Autodesk Inventor part; units mm, degrees
ref_plane "YZ Plane" through (0, 0, 0) normal (1, 0, 0) x (0, 1, 0)
ref_plane "XZ Plane" through (0, 0, 0) normal (0, 1, 0) x (-1, 0, 0)
ref_plane "XY Plane" through (0, 0, 0) normal (0, 0, 1) x (1, 0, 0)
sketch "Sketch1" plane through (0, 0, 0) normal (0, 1, 0) x (-1, 0, 0)
  arc A0 (-93.5462, 17.5) -> (-93.5462, -17.5) centre (-93.5462, 0) ccw
  arc A1 (-93.5462, 17.5) -> (-93.5462, -17.5) centre (-93.5462, 0) ccw
  line L0 (-68.5462, -17.5) -> (51.4538, -17.5)
  line L1 (51.4538, -17.5) -> (51.4538, 12.6842)
  line L2 (51.4538, 12.6842) -> (-68.5462, 12.6842)
  line L3 (-68.5462, 12.6842) -> (-68.5462, -17.5)
  line L4 (-68.5462, -17.5) -> (-93.5462, -17.5)
  arc A2 (76.4538, -17.5) -> (76.4538, 17.5) centre (76.4538, 0) ccw
  line L5 (51.4538, -17.5) -> (76.4538, -17.5)
  line L6 (76.4538, 17.5) -> (-93.5462, 17.5)
  point P0 (0, 0)
  dimension "d0" = 35
  dimension "d1" = 120
  dimension "d2" = 25
  dimension "d3" = 35
  dimension "d4" = 25
extrude "Extrusion1" add sketch "Sketch1" along normal blind 65 contours L6 A2 L5 L1 L2 L3 L4 A0
sketch "Sketch2" plane through (0, 65, 0) normal (0, 1, 0) x (1, 0, 0)
  arc A0 (-69.3673, -11.4905) -> (-75.5737, -13.4713) centre (-76.4538, 0) ccw
  arc A1 (92.6661, -13.4713) -> (86.972, -11.7911) centre (93.5462, 0) ccw
  line L0 (-51.4538, -12.6842) -> (-51.4538, 17.5)
  line L1 (68.5462, 17.5) -> (68.5462, -12.6842)
  line L2 (93.5462, -13.5) -> (68.5462, -12.6842)
  line L3 (-76.4538, -13.5) -> (-51.4538, -12.6842)
  line L4 (68.5462, -11.1899) -> (86.972, -11.7911)
  line L5 (-51.4538, -11.8536) -> (-69.3673, -11.4905)
  line L6 (-51.4538, -11.8536) -> (-51.4267, -12.6833)
  line L7 (68.5462, -11.1899) -> (68.5462, -12.6842)
  point P0 (0, 0)
  dimension "d7" = 27
  dimension "d8" = 27
  dimension "d9" = 25
  dimension "d10" = 25
extrude "Extrusion2" cut sketch "Sketch2" against normal blind 65 contours L5 L0 L3 A0 | L2 L1 L4 A1
sketch "Sketch4" plane through (0, 0, 0) normal (0, -1, 0) x (1, 0, 0)
  arc A0 (-76.4538, 13.5) -> (-69.3673, 11.4905) centre (-76.4538, 0) ccw
  arc A1 (-76.4538, 17.5) -> (-76.4538, -17.5) centre (-76.4538, 0) ccw
  arc A2 (93.5462, -17.5) -> (93.5462, 17.5) centre (93.5462, 0) ccw
  arc A3 (93.5462, -17.5) -> (93.5462, 17.5) centre (93.5462, 0) ccw
  line L0 (-76.4538, 17.5) -> (93.5462, 17.5)
  line L1 (-76.4538, 17.5) -> (93.5462, 17.5)
  line L2 (-51.4538, -17.5) -> (-76.4538, -17.5)
  line L3 (-76.4538, -17.5) -> (93.5462, -17.5)
  point P0 (0, 0)
extrude "Extrusion4" add sketch "Sketch4" along normal blind 5
sketch "Sketch5" plane through (0, 0, 0) normal (0, 1, 0) x (1, 0, 0)
  line L0 (-69.3673, -11.4905) -> (-51.4538, -11.8536)
  line L1 (68.5462, 17.5) -> (68.5462, -11.1899)
  line L2 (-51.4538, -11.8536) -> (68.5462, -11.8536)
  line L3 (68.5462, -11.8536) -> (68.5462, -8.8458)
  line L4 (68.5462, -8.8458) -> (-51.4538, -8.8458)
  line L5 (-51.4538, -8.8458) -> (-51.4538, -11.8536)
  point P0 (0, 0)
extrude "Extrusion5" add sketch "Sketch5" along normal blind 2
sketch "Sketch6" plane through (68.5462, 0, 8.8458) normal (0, 0, -1) x (-1, 0, 0)
  point P0 (68.5462, 0)
sketch "Sketch7" plane through (0, 0, 0) normal (0, 1, 0) x (1, 0, 0)
  line L0 (68.5462, -11.8536) -> (68.5462, -11.1899)
  line L1 (68.5462, -11.1899) -> (86.972, -11.7911)
  line L2 (68.5462, -11.8536) -> (86.972, -11.7911)
  line L3 (68.5462, -8.8458) -> (68.5462, -11.1899)
  line L4 (86.972, -11.7911) -> (68.5462, -11.1899)
  line L5 (68.5462, -11.1899) -> (68.5266, -11.7911)
  point P0 (0, 0)
extrude "Extrusion6" add sketch "Sketch7" along normal blind 65
sketch "Sketch8" plane through (-51.4538, 65, 11.8536) normal (1, 0, 0) x (0, 0, -1)
  line L0 (0, 0) -> (29.3536, 0)
  line L1 (0, 0) -> (4.0071, 0)
  line L2 (4.0071, 0) -> (4.0071, -2.0911)
  line L3 (4.0071, -2.0911) -> (0, -2.0911)
  line L4 (0, -2.0911) -> (0, 0)
  point P0 (11.8536, -65)
extrude "Extrusion7" add sketch "Sketch8" along normal blind 120
fillet "Fillet1" radius 0.5 1 edges at (-69.3673, 32.5, 11.4905)
fillet "Fillet2" radius 0.5 1 edges at (86.972, 32.5, 11.7911)
chamfer "Chamfer1" distance 1 angle 45 1 edges at (8.5462, 2, 8.8458)
chamfer "Chamfer2" distance 1 angle 45 1 edges at (8.5462, 62.9089, 7.8466)
sketch "Sketch9" plane through (0, 0, 0) normal (0, 1, 0) x (1, 0, 0)
  arc A0 (93.5462, -17.5) -> (93.5462, 17.5) centre (93.5462, 0) ccw
  line L0 (93.5462, 17.5) -> (68.5462, 17.5)
  line L1 (93.5462, 17.5) -> (93.5462, 17.5)
  circle A1 centre (93.5462, 0) radius 2
  line L2 (-76.4538, 17.5) -> (93.5462, 17.5)
  line L3 (-76.4538, -17.5) -> (93.5462, -17.5)
  circle A2 centre (-76.4538, 0) radius 2
  point P0 (0, 0)
  dimension "d39" = 4
  dimension "d40" = 4
extrude "Extrusion8" add sketch "Sketch9" along normal blind 5
fillet "Fillet3" radius 0.5 2 edges at (91.5462, 5, 0) (-78.4538, 5, 0)
sketch "Sketch10" plane through (-51.4538, 65, -17.5) normal (0, 0, -1) x (-1, 0, 0)
  circle A0 centre (-125, -5) radius 1.75
  circle A1 centre (-125, -60) radius 1.75
  line L0 (25, -70) -> (-145, -70)
  line L1 (-120, -65) -> (-120, 0)
  line L2 (-145, 0) -> (-120, 0)
  circle A2 centre (5, -60) radius 1.75
  circle A3 centre (5, -5) radius 1.75
  line L3 (0, -65) -> (0, 0)
  line L4 (0, 0) -> (25, 0)
  point P0 (-51.4538, -65)
  dimension "d44" = 3.5
  dimension "d45" = 3.5
  dimension "d46" = 10
  dimension "d47" = 5
  dimension "d48" = 5
  dimension "d49" = 3.5
  dimension "d50" = 3.5
  dimension "d51" = 5
  dimension "d52" = 5
  dimension "d53" = 5
  dimension "d54" = 10
extrude "Extrusion9" cut sketch "Sketch10" against normal blind 10
sketch "Sketch11" plane through (0, 65, 0) normal (0, 1, 0) x (1, 0, 0)
  point P0 (0, 0)
sketch "Sketch12" plane through (0, 65, 0) normal (0, 1, 0) x (1, 0, 0)
  circle A0 centre (73.5462, -2.5) radius 2
  circle A1 centre (-56.4538, -2.5) radius 2
  line L0 (68.5462, 17.5) -> (68.5462, -7.8466)
  line L1 (93.5462, 17.5) -> (68.5462, 17.5)
  line L2 (-51.4538, -7.8466) -> (-51.4538, 17.5)
  arc A2 (93.5462, -17.5) -> (93.5462, 17.5) centre (93.5462, 0) ccw
  point P0 (0, 0)
  dimension "d57" = 4
  dimension "d58" = 4
  dimension "d59" = 5
  dimension "d60" = 20
  dimension "d61" = 5
  dimension "d62" = 20
extrude "Extrusion10" cut sketch "Sketch12" against normal blind 10
sketch "Sketch13" plane through (0, 65, 0) normal (0, 1, 0) x (1, 0, 0)
  circle A0 centre (93.5462, 0) radius 1.5
  arc A1 (93.5462, -16.75) -> (93.5462, 16.75) centre (93.5462, 0) ccw
  circle A2 centre (93.5462, 0) radius 2
  arc A3 (93.5462, -15.75) -> (93.5462, 15.75) centre (93.5462, 0) ccw
  circle A4 centre (-76.4538, 0) radius 1.5
  arc A5 (-76.4538, 16.75) -> (-76.4538, -16.75) centre (-76.4538, 0) ccw
  arc A6 (-76.4538, 15.75) -> (-76.4538, -15.75) centre (-76.4538, 0) ccw
  line L0 (93.5462, -16.75) -> (-76.4538, -16.75)
  line L1 (-76.4538, -15.75) -> (93.5462, -15.75)
  line L2 (-76.4538, 15.75) -> (-55.2204, 15.75)
  line L3 (-55.2204, 15.75) -> (-55.2204, 16.75)
  line L4 (-55.2204, 16.75) -> (-76.4538, 16.75)
  line L5 (93.5462, 15.75) -> (71.4067, 15.75)
  line L6 (71.4067, 15.75) -> (71.4067, 16.75)
  line L7 (71.4067, 16.75) -> (93.5462, 16.75)
  point P0 (0, 0)
  dimension "d65" = 33.5
  dimension "d66" = 31.5
  dimension "d67" = 33.5
  dimension "d68" = 31.5
extrude "Extrusion11" add sketch "Sketch13" along normal blind 2 contours L0 A5 L4 L3 L2 A6 L1 A3 L5 L6 L7 A1
sketch "Sketch14" plane through (-51.4538, 65, -17.5) normal (0, 0, -1) x (-1, 0, 0)
  point P0 (-51.4538, -65)
properties part number "C-PAN"
The listing builds one solid part. Answer for the finished solid, in the listing's coordinates (mm). A direction names the side the tool comes from. Give positions to 0.01 mm unless a question says otherwise; leave off trailing zeros. Write each loop counter-clockwise with the first axis right and the second up, starting at its lowest first coordinate (ties: lowest second). Pieces come first, ordered by that corner, then holes. Notation, with made-up numbers: (48.5, 19.5) - (68.5, 19.5) arc R13 ccw to (68.5, 23.5) - close; hole circle Ø4 at (11, 63). An arc over 180 degrees is marked (long way). Use one line per item in the form item = value. Start each with the question number.
1) Find section A-A on x = 24.5. Determine the outline of the cut face in (y, z).
2) Find section D-D on x = 77.5. Determine the outline of the cut face in (y, z), plus the area to 3 significant figures.
3) The mould has two halves that part along X. Classify faces 1 (the face through (71.55, 60.07, 2.41)), 2 (the face through (-56, 5, -7.5)), 3 (the face through (-93.2, 66, 0.4)), 4 (the face through (9, -1, -17.5)): pulls with the +X half, pulls with the -X half, needs draft (parallel to the pull), parting line crosses it, or undercut.
4) Find section C-C on y = 12.5. Determine the outline of the cut face in (x, z).
5) Consider line 1 along Z through (x, y) = (-65, 60); line 2 along X through (y, z) = (32.5, -4); line 3 along Z through (x, y) = (-77, 24). Determine where each line is inside the solid, lowest interval first. Write a range as from..to.
6) Find section B-B on z = -11.5. Determine the outline of the cut face in (x, y).
7) Flat-ended cylindrical pins translate along their axes: pin 1 Ø1 at (y, z) = (16, -5) entering from -X; pin 2 Ø6 at (x, y) = (58, 40) entering from -Z; pin 3 Ø1.8 at (x, y) = (73, 60) entering from -Z; pin 4 Ø4.5 at (x, y) = (-56.45, 5) entering from -Z. Find the tip coordinate at first contact, or state that the pin passes through.
8) A tool of negligible diameter and unlimited length cuts with its end or side. For faces 5 (the face through (73.926, 3.292, -12.57)), 6 (the face through (-93.95, 30.49, -0.38)), 7 (the face through (-92.2, 66, 0.3)), from which of +Z, -Z, +X, -X, +Y, -Y can it reach the whole face along a straight path? Write none if from no direction.
Geometry results:
q1.outline = (-5, -17.5) - (0, -17.5) - (0, 8.85) - (1, 8.85) - (2, 9.85) - (2, 11.85) - (0, 11.85) - (0, 12.68) - (65, 12.68) - (65, 15.75) - (67, 15.75) - (67, 16.75) - (65, 16.75) - (65, 17.5) - (-5, 17.5) - close; (62.91, 8.85) - (63.91, 7.85) - (65, 7.85) - (65, 11.85) - (62.91, 11.85) - close
q2.outline = (-5, -17.5) - (65, -17.5) - (65, -16.75) - (67, -16.75) - (67, -15.75) - (65, -15.75) - (65, 11.82) - (0, 11.82) - (0, 12.98) - (65, 12.98) - (65, 15.75) - (67, 15.75) - (67, 16.75) - (65, 16.75) - (65, 17.5) - (-5, 17.5) - close
q2.area = 2,380 mm2
q3.face_1 = undercut
q3.face_2 = undercut
q3.face_3 = pulls with the -X half
q3.face_4 = needs draft
q4.outline = (-76.45, -17.5) - (-51.45, -17.5) - (-51.45, 11.85) - (-67.83, 11.52) arc R0.5 ccw to (-68.13, 10.63) arc R13.5 cw (long way) to (-76.45, 13.5) - (-51.45, 12.68) - (68.55, 12.68) - (93.55, 13.5) arc R13.5 cw (long way) to (85.57, 10.89) arc R0.5 ccw to (85.28, 11.8) - (68.55, 11.85) - (68.55, -17.5) - (93.55, -17.5) arc R17.5 ccw to (93.55, 17.5) - (-76.45, 17.5) arc R17.5 ccw to start
q5.line_1 = -17.5..-7.15, 7.15..11.58, 13.13..17.5
q5.line_2 = -93.49..-89.35, -63.56..-51.45, 68.55..80.65, 106.44..110.58
q5.line_3 = -17.49..-13.49, 13.49..17.49
q6.outline = (-89.64, -5) - (106.74, -5) - (106.74, 65) - (105.72, 65) - (105.72, 67) - (104.31, 67) - (104.31, 65) - (100.62, 65) - (100.62, 0) - (86.48, 0) - (86.48, 65) - (68.55, 65) - (68.55, 0) - (-51.45, 0) - (-51.45, 65) - (-69.38, 65) - (-69.38, 0) - (-83.52, 0) - (-83.52, 65) - (-87.22, 65) - (-87.22, 67) - (-88.63, 67) - (-88.63, 65) - (-89.64, 65) - close; hole circle Ø3.5 at (-56.45, 5); hole circle Ø3.5 at (-56.45, 60); hole circle Ø3.5 at (73.55, 5); hole circle Ø3.5 at (73.55, 60)
q7.pin_1 = -93.37
q7.pin_2 = 12.68
q7.pin_3 = -7.5
q7.pin_4 = -17.5
q8.face_5 = -Z
q8.face_6 = -X, +Y, -Y
q8.face_7 = +Y
